Answer from the drawing. Dimensions are ordinates in mm from the lowest x, y and z of the part. Round coordinates to 2 decimals unless told otherwise and drop trailing zeros. Write each loop counter-clockwise with the first axis right and the second up, starting at its lowest first coordinate (ties: lowest second). Pieces come first, ordered by that corner, then holes. Notation, with made-up numbers: M 41.25,77 L 85.25,77 A10 ccw 85.25,81 Z; hole C -4.75,-33.5 d7. An arc over 180 degrees is marked long. One line per item, written item: value. Start each with the question number.
(1) Section A-A (x = 7.65) is taken. Determine the outline of the cut face in (y, z).
(2) Given P1, Ø6, axis at y = 4, z = 2, coming from the -X side; P2, Ø6, axis at x = 13.5, z = 1.5, coming from the -Y side; P3, Ø3, axis at x = 4.5, y = 8.5, coming from the +Z side, each flat-ended and moving along its own axis, determine where each tip first touches the part or whether it passes through.
(3) Consider probe 1 along Y at (x, z) = (7.65, 3.25); probe 2 along X at (y, z) = (8.75, 4.75) (1 decimal). Determine where each line is inside the solid, lowest interval first.
(4) Section C-C (z = 4) is taken. Determine the outline of the cut face in (x, y).
(5) For a pull along Y with two mould halves and no side action, classify the marked faces 1, 2 and 3 as released by +Y, released by -Y, zero draft, split by the parting line, or undercut.
(6) Section D-D (x = 14) is taken. Determine the outline of the cut face in (y, z).
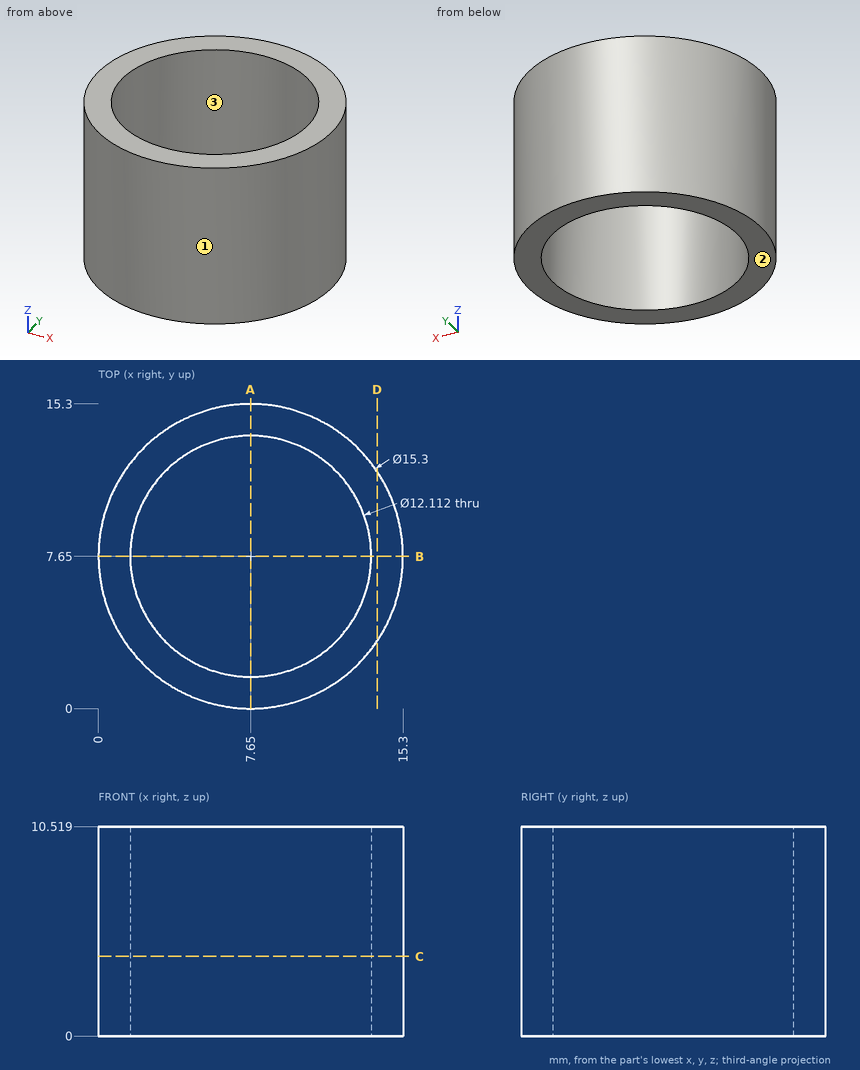
Recorded:
1. outline: M 0,0 L 1.59,0 L 1.59,10.52 L 0,10.52 Z; M 13.71,0 L 15.3,0 L 15.3,10.52 L 13.71,10.52 Z
2. P1: stops at x = 0.03
2. P2: stops at y = 0.55
2. P3: passes through
3. probe 1: y = 0 to 1.59, 13.71 to 15.3
3. probe 2: x = 0.1 to 1.7, 13.6 to 15.2
4. outline: C 7.65,7.65 d15.3; hole C 7.65,7.65 d12.11
5. face 1: split by the parting line
5. face 2: zero draft
5. face 3: undercut
6. outline: M 3.38,0 L 11.92,0 L 11.92,10.52 L 3.38,10.52 Z
